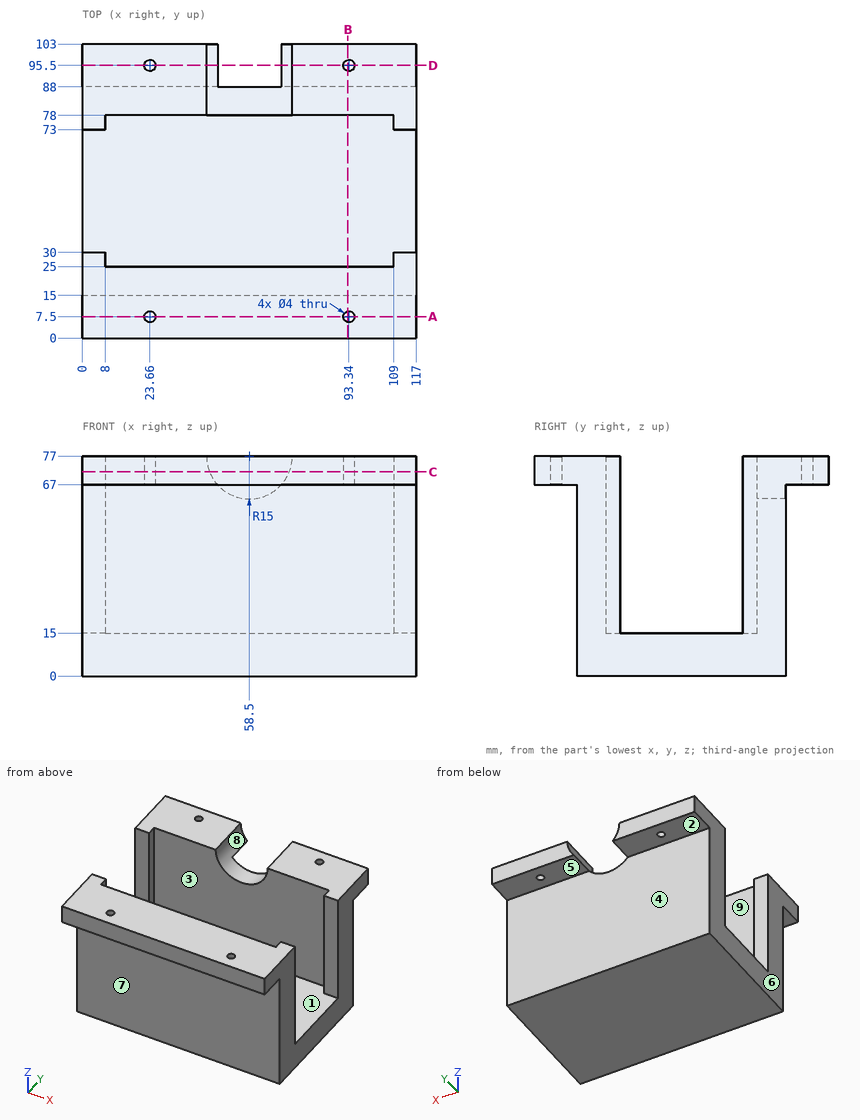
Input: dimensioned drawing with shaded views. Units: mm. Origin: part minimum x, y, z. A direction names the side the tool comes from. Round coordinates to 2 decimals unless told otherwise and drop trailing zeros. Loops run counter-clockwise (first coordinate to the right, second up) from the corner with the lowest first, then second, coordinate; pieces in that order, holes last. Notation, with made-up numbers: (-29.5, 36.5) -> (10.5, 36.5) arc R30 cw to (10.5, 75.5) -> close; hole circle Ø6 at (18.5, 29.5). An arc over 180 degrees is marked (long way). One line per item, written item: value.
(1) Material intervals for line 1 (Y direction, x = 55, z = 58); line 2 (X direction, y = 7, z = 74); line 3 (X direction, y = 95.5, z = 70.25) (1 decimal), sorted ascending. Write a range as [from, to].
Geometry check:
line 1: [15, 25], [78, 88]
line 2: [0, 21.72], [25.6, 91.4], [95.28, 117]
line 3: [0, 21.7], [25.7, 45.1], [71.9, 91.3], [95.3, 117]
(2) Section B-B (x = 93). Return the cut outline in (y, z).
Geometry check:
outline: (0, 67) -> (5.53, 67) -> (5.53, 77) -> (0, 77) -> close; (9.47, 67) -> (15, 67) -> (15, 0) -> (88, 0) -> (88, 67) -> (93.53, 67) -> (93.53, 77) -> (78, 77) -> (78, 15) -> (25, 15) -> (25, 77) -> (9.47, 77) -> close; (97.47, 67) -> (103, 67) -> (103, 77) -> (97.47, 77) -> close
(3) Mould query, pull axis Y, two halves, no side actions, for the marked faces 1, 2, 3 and 4. Classes: pulls with the +Y half, pulls with the -Y half, needs draft (parallel to the pull), parting line crosses it, or undercut.
Geometry check:
face 1: undercut
face 2: needs draft
face 3: undercut
face 4: pulls with the +Y half
(4) Section D-D (y = 95.5). Return the cut outline in (x, z), plus the area to 3 significant figures.
Geometry check:
outline: (0, 67) -> (21.66, 67) -> (21.66, 77) -> (0, 77) -> close; (25.66, 67) -> (47.32, 67) arc R15 cw to (43.5, 77) -> (25.66, 77) -> close; (69.68, 67) -> (91.34, 67) -> (91.34, 77) -> (73.5, 77) arc R15 cw to start; (95.34, 67) -> (117, 67) -> (117, 77) -> (95.34, 77) -> close
area: 814 mm2
(5) Section A-A (y = 7.5). Return the cut outline in (x, z), plus the area to 3 significant figures.
Geometry check:
outline: (0, 67) -> (21.66, 67) -> (21.66, 77) -> (0, 77) -> close; (25.66, 67) -> (91.34, 67) -> (91.34, 77) -> (25.66, 77) -> close; (95.34, 67) -> (117, 67) -> (117, 77) -> (95.34, 77) -> close
area: 1,090 mm2
(6) Pin query (flat end, axial travel): pin 1 (20 mm diameter, centred on x = 56.5, z = 26.5, fed in from +Y); pin 2 (4.5 mm diameter, centred on x = 29.5, y = 5.5, fed in from -Z); pin 3 (3 mm diameter, centred on x = 93.34, y = 95.5, fed in from -Z); pin 4 (6.5 mm diameter, centred on x = 4.5, z = 45, fed in from -Y). Return the tip coordinate at first contact, or that it passes through.
Geometry check:
pin 1: y = 88
pin 2: z = 67
pin 3: through
pin 4: y = 15
(7) Set-up query: the marked faces 5, 6, 7, 8 and 9. Return all of +Z, -Z, +X, -X, +Y, -Y with unobstructed straight access to the full face (end or side cutting, diameter ignored); none if empty.
Geometry check:
face 5: -Z, +X, -X, +Y
face 6: +Z, -Z, -X, +Y, -Y
face 7: -Z, +X, -X, -Y
face 8: +Z, +Y
face 9: +Z
(8) Section C-C (z = 71.5). Return the cut outline in (x, y) (1 decimal).
Geometry check:
outline: (0, 0) -> (117, 0) -> (117, 30) -> (109, 30) -> (109, 25) -> (8, 25) -> (8, 30) -> (0, 30) -> close; (0, 73) -> (8, 73) -> (8, 78) -> (44.5, 78) -> (44.5, 103) -> (0, 103) -> close; (72.5, 78) -> (109, 78) -> (109, 73) -> (117, 73) -> (117, 103) -> (72.5, 103) -> close; hole circle Ø4 at (23.7, 7.5); hole circle Ø4 at (23.7, 95.5); hole circle Ø4 at (93.3, 7.5); hole circle Ø4 at (93.3, 95.5)
